Geometry check sheet. Reference: the model listing, model coordinates, mm. Coordinates: 2 decimals unless noted, no trailing zeros. Loops run counter-clockwise (first coordinate to the right, second up) from the corner with the lowest first, then second, coordinate; pieces in that order, holes last. Notation, with made-up numbers: (26.25, -37) - (57.25, -37) arc R9 cw to (57.25, -22) - close; hole circle Ø7 at (41, -10). An arc over 180 degrees is marked (long way). One line per item, written item: value.
from build123d import *

# Parameters (mm, degrees)
SKETCH1_W           = 120
SKETCH1_H           = 105
BOSS_EXTRUDE1_DEPTH = 2
SKETCH2_W           = 24.020633768
SKETCH2_H           = 13.604733883
SKETCH2_W_2         = 15.976853837
SKETCH2_H_2         = 7.633913726
SKETCH2_W_3         = 9.287125415
SKETCH2_H_3         = 5.814380322
SKETCH2_W_4         = 11.648356386
SKETCH2_W_5         = 21.267599873
SKETCH2_H_4         = 7.189917071
BOSS_EXTRUDE2_DEPTH = 1


with BuildPart() as part:
    # Sketch1 → Boss-Extrude1 (new body)
    with BuildSketch(Plane.XY):
        Rectangle(SKETCH1_W, SKETCH1_H)
    extrude(amount=BOSS_EXTRUDE1_DEPTH)

    # Sketch2 → Boss-Extrude2 (add)
    with BuildSketch(Plane.XY.offset(2)):
        with Locations((-26.865959822, -22.784123417)):
            Rectangle(SKETCH2_W, SKETCH2_H)
        with Locations((30.883941206, -26.60108028)):
            Rectangle(SKETCH2_W_2, SKETCH2_H_2)
        with Locations((-31.509522529, 21.57302436)):
            Rectangle(SKETCH2_W_3, SKETCH2_H_3)
        with Locations((30.883941206, 21.57302436)):
            Rectangle(SKETCH2_W_4, SKETCH2_H_3)
        with Locations((-44.38112644, -46.052934011)):
            Rectangle(SKETCH2_W_5, SKETCH2_H_4)
    extrude(amount=BOSS_EXTRUDE2_DEPTH)


solid = part.part
(1) Cross-section at B-B on x = 32.5. Record the cut outline in (y, z), and give its area (3 significant figures).
Reply:
outline: (-52.5, 0) - (52.5, 0) - (52.5, 2) - (24.48, 2) - (24.48, 3) - (18.67, 3) - (18.67, 2) - (-22.78, 2) - (-22.78, 3) - (-30.42, 3) - (-30.42, 2) - (-52.5, 2) - close
area: 223 mm2
(2) Material ranges on probe 1 along Y at (x, z) = (-34.5, 2.85); probe 2 along Z at (x, y) = (18, 30); probe 3 along Y at (x, z) = (-41.5, 2.65), recorded low to high. Write a range as from..to.
Reply:
probe 1: -49.65..-42.46, -29.59..-15.98, 18.67..24.48
probe 2: 0..2
probe 3: -49.65..-42.46
(3) Cross-section at D-D on x = -3. Record the cut outline in (y, z), and give its area (3 significant figures).
Reply:
outline: (-52.5, 0) - (52.5, 0) - (52.5, 2) - (-52.5, 2) - close
area: 210 mm2
(4) Go/stop test with flat-tipped pins: pin 1 Ø4 at (x, y) = (15.5, -13) entering from +Z; pin 2 Ø0.8 at (x, z) = (-41.5, 2.5) entering from -Y; pin 3 Ø0.8 at (x, z) = (33, 2.5) entering from +Y. Record where each tip stops, or that it passes through.
Reply:
pin 1: z = 2
pin 2: y = -49.65
pin 3: y = 24.48
(5) Cross-section at A-A on y = -27. Record the cut outline in (x, z), and give its area (3 significant figures).
Reply:
outline: (-60, 0) - (60, 0) - (60, 2) - (38.87, 2) - (38.87, 3) - (22.9, 3) - (22.9, 2) - (-14.86, 2) - (-14.86, 3) - (-38.88, 3) - (-38.88, 2) - (-60, 2) - close
area: 280 mm2
(6) Cross-section at C-C on y = -2.5. Record the cut outline in (x, z).
Reply:
outline: (-60, 0) - (60, 0) - (60, 2) - (-60, 2) - close
